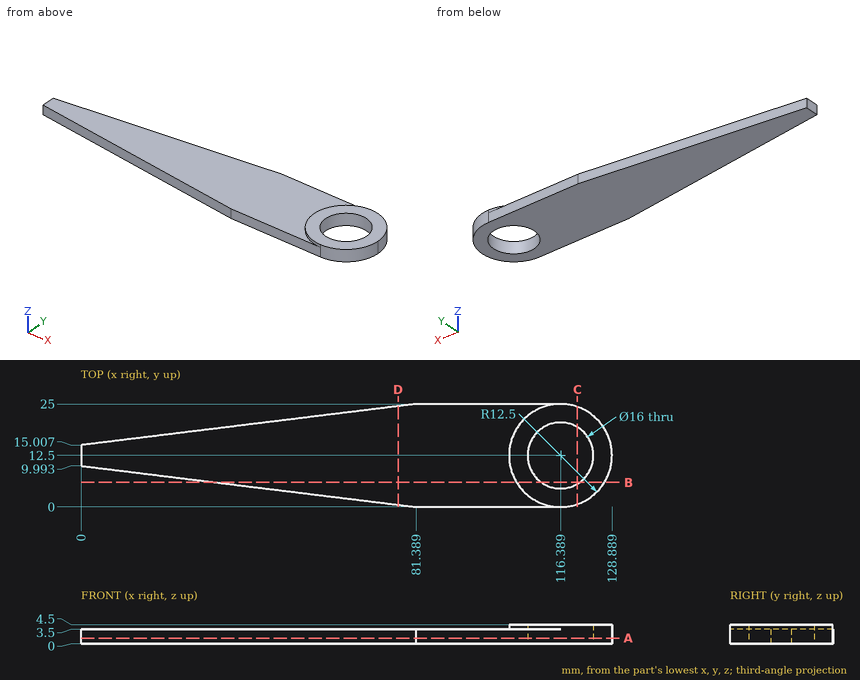
Job drawing, mm, ordinate dimensions from the low corner. One solid piece. Coordinates: 2 decimals unless noted, no trailing zeros. Loops run counter-clockwise (first coordinate to the right, second up) from the corner with the lowest first, then second, coordinate; pieces in that order, holes last. Notation, with made-up numbers: (12.5, 63) - (37.5, 63) arc R15 ccw to (37.5, 74) - close; hole circle Ø2 at (-39.5, -12.75). An arc over 180 degrees is marked (long way). Answer as a JSON object with one key per item and string values. Group by question number.
(1) Flat gauge pin, fed straight in: pin 1 (1 mm diameter, centred on x = 54, z = 1, fed in from +Y). Where does the tip first touch, or does it go through?
(2) Cut at C-C (x = 120.5). Give the cut face in (y, z) (1 decimal).
(3) Cut at B-B (y = 6). Give the cut face in (x, z) (1 decimal).
(4) Cut at A-A (z = 1.3). Give the cut face in (x, y).
(5) Cut at D-D (x = 77). Give the cut face in (y, z).
(6) Probe line 1 along Z through (x, y) = (6, 10.75); line 2 along Y through (x, z) = (73, 2.2); line 3 along Y through (x, z) = (67, 2.4). List the from-to ranges inside material, lowest first.
Geometry says:
{
 "1": {"pin 1": "stops at y = 21.7"},
 "2": {"outline": "(0.7, 0) - (5.6, 0) - (5.6, 4.5) - (0.7, 4.5) - close; (19.4, 0) - (24.3, 0) - (24.3, 4.5) - (19.4, 4.5) - close"},
 "3": {"outline": "(32.5, 0) - (111.7, 0) - (111.7, 4.5) - (105.7, 4.5) - (105.7, 3.5) - (32.5, 3.5) - close; (121.1, 0) - (127.1, 0) - (127.1, 4.5) - (121.1, 4.5) - close"},
 "4": {"outline": "(0, 9.99) - (81.39, 0) - (116.39, 0) arc R12.5 ccw to (128.89, 12.5) arc R12.5 ccw to (116.39, 25) - (81.39, 25) - (0, 15.01) - close; hole circle Ø16 at (116.39, 12.5)"},
 "5": {"outline": "(0.54, 0) - (24.46, 0) - (24.46, 3.5) - (0.54, 3.5) - close"},
 "6": {"line 1": "z = 0 to 3.5", "line 2": "y = 1.03 to 23.97", "line 3": "y = 1.77 to 23.23"}
}
